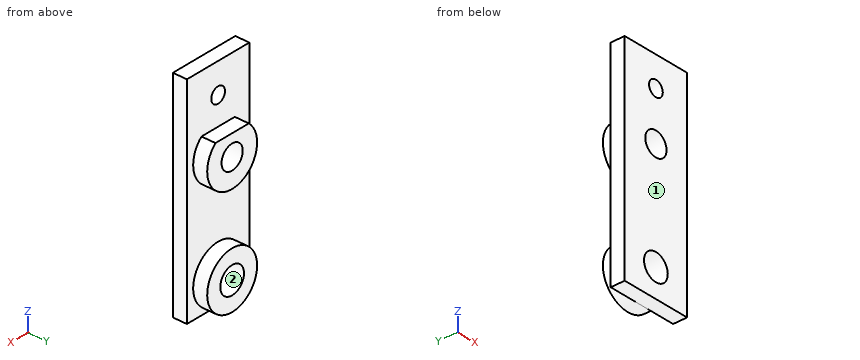
from build123d import *

# Parameters (mm, degrees)
SKETCH_1_W          = 25
SKETCH_1_H          = 76.5
SKETCH_1_R          = 4.75
SKETCH_1_R_2        = 4.25
EXTRUDE_1_DEPTH     = 5
SKETCH_2_R          = 2.75
CUT_EXTRUDE_1_DEPTH = 64.300866763
SKETCH_3_R          = 10
SKETCH_3_R_2        = 4.75
SKETCH_3_R_3        = 4.25
EXTRUDE_2_DEPTH     = 5


with BuildPart() as part:
    # 草图1 → 凸台-拉伸1 (new body)
    with BuildSketch(Plane(origin=(0, 0, 0), x_dir=(1, 0, 0), z_dir=(0, 1, 0))):
        with Locations((-26.981132075, -10.976415094)):
            Rectangle(SKETCH_1_W, SKETCH_1_H)
        with Locations(Location((-26.981132075, 17.273584906, 0), (0, 0, 270))):
            Circle(SKETCH_1_R, mode=Mode.SUBTRACT)
        with Locations(Location((-26.981132075, -21.226415094, 0), (0, 0, 270))):
            Circle(SKETCH_1_R_2, mode=Mode.SUBTRACT)
    extrude(amount=EXTRUDE_1_DEPTH)

    # 草图2 → 切除-拉伸1 (cut, through all)
    with BuildSketch(Plane(origin=(0, 0, 0), x_dir=(-1, 0, 0), z_dir=(0, -1, 0))):
        with Locations(Location((26.981132075, -38.580008519, 0), (0, 0, 90))):
            Circle(SKETCH_2_R)
    extrude(amount=-CUT_EXTRUDE_1_DEPTH, mode=Mode.SUBTRACT)

    # 草图3 → 凸台-拉伸2 (add)
    # profile 1 of 2: a face of its own
    with BuildSketch(Plane(origin=(0, 5, 0), x_dir=(1, 0, 0), z_dir=(0, 1, 0))):
        with Locations(Location((-26.981132075, 17.273584906, 0), (0, 0, 90))):
            Circle(SKETCH_3_R)
        with Locations(Location((-26.981132075, 17.273584906, 0), (0, 0, 270))):
            Circle(SKETCH_3_R_2, mode=Mode.SUBTRACT)
    # profile 2 of 2: a face of its own
    with BuildSketch(Plane(origin=(0, 5, 0), x_dir=(1, 0, 0), z_dir=(0, 1, 0))):
        with BuildLine():
            Line((-33.65845117, -28.670433479), (-20.303812981, -28.670433479))
            ThreePointArc((-20.303812981, -28.670433479), (-26.981132075, -11.226415094), (-33.65845117, -28.670433479))
        make_face()
        with Locations(Location((-26.981132075, -21.226415094, 0), (0, 0, 270))):
            Circle(SKETCH_3_R_3, mode=Mode.SUBTRACT)
    extrude(amount=EXTRUDE_2_DEPTH)


solid = part.part
The listing builds one solid part. Answer for the finished solid, in the listing's coordinates (mm). Face numbers are marked on the shaded views. Coordinates: 2 decimals unless noted, no trailing zeros. Order: outer loops, then holes, each group sorted by start corner. A loop starts at its lowest first (then second) coordinate and runs counter-clockwise, first axis right, second up. Notation, with made-up numbers: (6.25, 51.25) -> (46.25, 51.25) arc R21 ccw to (46.25, 56.25) -> close; hole circle Ø2 at (27.5, 88). An arc over 180 degrees is marked (long way). Answer in a Markdown table with one row per item. Add a question column.
Item 1: Determine the mould class of the marked faces 1 and 2 for opening direction X: +X half, -X half, draft (parallel to the pull), parting line (faces both ways), or undercut.
Item 2: Find section A-A (y = 7.25). Write down the section's boundary in (x, z), then the cut area to 3 significant figures.
Item 3: Find section D-D (y = 1.25). Write down the section's boundary in (x, z), then the cut area to 3 significant figures.
Item 4: Find section B-B (z = 38.5). Write down the section's boundary in (x, y).
Item 5: Find section C-C (x = -30.5). Write down the section's boundary in (y, z), then the cut area to 3 significant figures.
Item 6: Each of these flat-tipped pins is pushed along its axis until it touches: P1, Ø10, axis at x = -36.5, z = 41, coming from the +Y side; P2, Ø5.5, axis at x = -30.5, y = 8, coming from the +Z side; P3, Ø4, axis at y = 9, z = 17.5, coming from the -X side. Where does it stop, or does it pass through?
Item 7: Find the intervals of material crossed by L1, parallel to Z at x = -26.75, y = 5.5; L2, parallel to Z at x = -24, y = 4.25; L3, parallel to Z at x = -25.75, y = 9.75, in increasing order. Write a range as from..to.
Result set:
| question | item | result |
|---|---|---|
| 1 | face 1 | draft |
| 1 | face 2 | undercut |
| 2 | outline | circle Ø20 at (-26.98, -17.27); (-33.66, 28.67) arc R10 ccw (long way) to (-20.3, 28.67) -> close; hole circle Ø9.5 at (-26.98, -17.27); hole circle Ø8.5 at (-26.98, 21.23) |
| 2 | area | 477 mm² |
| 3 | outline | (-39.48, -27.27) -> (-14.48, -27.27) -> (-14.48, 49.23) -> (-39.48, 49.23) -> close; hole circle Ø9.5 at (-26.98, -17.27); hole circle Ø8.5 at (-26.98, 21.23); hole circle Ø5.5 at (-26.98, 38.58) |
| 3 | area | 1,760 mm² |
| 4 | outline | (-39.48, 0) -> (-29.73, 0) -> (-29.73, 5) -> (-39.48, 5) -> close; (-24.23, 0) -> (-14.48, 0) -> (-14.48, 5) -> (-24.23, 5) -> close |
| 5 | outline | (0, -27.27) -> (5, -27.27) -> (5, -26.63) -> (10, -26.63) -> (10, -20.46) -> (0, -20.46) -> close; (0, -14.08) -> (10, -14.08) -> (10, -7.91) -> (5, -7.91) -> (5, 11.87) -> (10, 11.87) -> (10, 18.84) -> (0, 18.84) -> close; (0, 23.61) -> (10, 23.61) -> (10, 28.67) -> (5, 28.67) -> (5, 49.23) -> (0, 49.23) -> close |
| 5 | area | 449 mm² |
| 6 | P1 | stops at y = 5 |
| 6 | P2 | stops at z = 28.67 |
| 6 | P3 | stops at x = -36.83 |
| 7 | L1 | z = -27.27..-22.02, -12.53..-7.28, 11.23..16.98, 25.47..28.67 |
| 7 | L2 | z = -27.27..-20.97, -13.58..18.2, 24.26..49.23 |
| 7 | L3 | z = -27.2..-21.86, -12.69..-7.35, 11.3..17.16, 25.29..28.67 |
